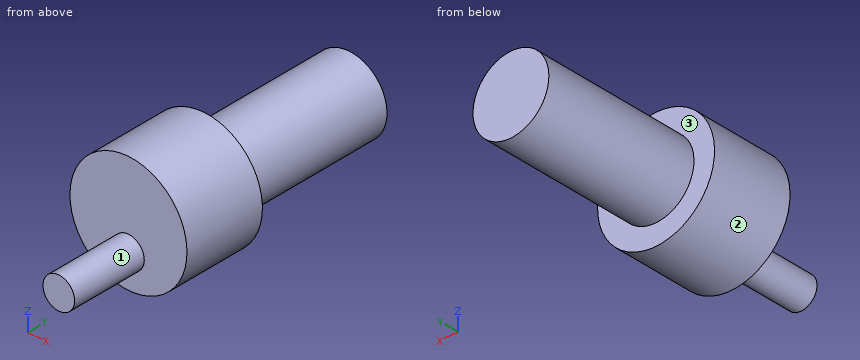
from build123d import *

# Parameters (mm, degrees)
ESBO_O1_R                = 18.5
RESSALTO_EXTRUS_O1_DEPTH = 100
CORTE_EXTRUS_O1_START    = -50
ESBO_O2_R                = 18.5
ESBO_O2_R_2              = 12
CORTE_EXTRUS_O1_DEPTH    = 50
ESBO_O3_R                = 18.5
ESBO_O3_R_2              = 5
CORTE_EXTRUS_O2_DEPTH    = 24


with BuildPart() as part:
    # Esboço1 → Ressalto-extrusão1 (new body)
    with BuildSketch(Plane(origin=(0, 0, 0), x_dir=(1, 0, 0), z_dir=(0, 1, 0))):
        with Locations(Location((0, 0, 0), (0, 0, 270))):
            Circle(ESBO_O1_R)
    extrude(amount=RESSALTO_EXTRUS_O1_DEPTH)

    # Esboço2 → Corte-extrusão1 (cut)
    with BuildSketch(Plane(origin=(0, 100, 0), x_dir=(1, 0, 0), z_dir=(0, 1, 0)).offset(CORTE_EXTRUS_O1_START)):
        with Locations(Location((0, 0, 0), (0, 0, 270))):
            Circle(ESBO_O2_R)
        with Locations(Location((0, 0, 0), (0, 0, 270))):
            Circle(ESBO_O2_R_2, mode=Mode.SUBTRACT)
    extrude(amount=CORTE_EXTRUS_O1_DEPTH, mode=Mode.SUBTRACT)

    # Esboço3 → Corte-extrusão2 (cut)
    with BuildSketch(Plane(origin=(0, 0, 0), x_dir=(-1, 0, 0), z_dir=(0, -1, 0))):
        with Locations(Location((0, 0, 0), (0, 0, 90))):
            Circle(ESBO_O3_R)
        with Locations(Location((0, 8, 0), (0, 0, 90))):
            Circle(ESBO_O3_R_2, mode=Mode.SUBTRACT)
    extrude(amount=-CORTE_EXTRUS_O2_DEPTH, mode=Mode.SUBTRACT)


solid = part.part
Can you work these out from the model? Positions are in its coordinate system, mm. Face numbers are marked on the shaded views. A direction names the side the tool comes from. Coordinates: 2 decimals unless noted, no trailing zeros. Loops run counter-clockwise (first coordinate to the right, second up) from the corner with the lowest first, then second, coordinate; pieces in that order, holes last. Notation, with made-up numbers: M -9,52.5 L 7,52.5 A25 ccw 7,81.5 Z; hole C 73.5,34 d10. An arc over 180 degrees is marked long. Answer as CSV lines item,"result". Start each with the question number.
1. Suppose I cut it at B-B, the plane x = 0. List the corners of the cut face in (y, z) for me.
2. Suppose I cut it at A-A, the plane z = 0. List the corners of the cut face in (x, y) for me, plus the area to 3 significant figures.
3. Suppose I cut it at C-C, the plane y = 15.5. List the corners of the cut face in (x, z) for me.
4. For the marked faces 1, 2 and 3, which set-ups out of +Z, -Z, +X, -X, +Y, -Y let a thin tool reach every point of the face, with its end or its side?
5. For pin 1 Ø8 at (x, y) = (1, 18.5) entering from -Z; pin 2 Ø4 at (y, z) = (65, 13) entering from -X; pin 3 Ø1 at (y, z) = (56.5, -5.5) entering from +X, each with a flat end and sliding along its axis, tell me the tip position at first contact or that it passes through.
6. Suppose I cut it at D-D, the plane z = -8. List the corners of the cut face in (x, y) for me.
7. If I drill on probe 1 along Y at (x, z) = (2.5, 11.5); probe 2 along Y at (x, z) = (4.5, 12); probe 3 along X at (y, z) = (45, 9.5), over which ranges is the centre line in solid material (lowest first)? Write a range as [from, to].
Output:
1,outline,"M 0,-13 L 24,-13 L 24,-18.5 L 50,-18.5 L 50,-12 L 100,-12 L 100,12 L 50,12 L 50,18.5 L 24,18.5 L 24,-3 L 0,-3 Z"
2,outline,"M -18.5,24 L 18.5,24 L 18.5,50 L 12,50 L 12,100 L -12,100 L -12,50 L -18.5,50 Z"
2,area,"2,160 mm^2"
3,outline,"C 0,-8 d10"
4,face 1,"-Y"
4,face 2,"+Y, -Y"
4,face 3,"+Y"
5,pin 1,"stops at z = -13"
5,pin 2,"stops at x = -4.8"
5,pin 3,"stops at x = 10.91"
6,outline,"M -16.68,24 L -5,24 L -5,0 L 5,0 L 5,24 L 16.68,24 L 16.68,50 L 8.94,50 L 8.94,100 L -8.94,100 L -8.94,50 L -16.68,50 Z"
7,probe 1,"y = [24, 100]"
7,probe 2,"y = [24, 50]"
7,probe 3,"x = [-15.87, 15.87]"
